from build123d import *

# Parameters (mm, degrees)
SKETCH_1_R      = 3
SKETCH_1_R_2    = 5
EXTRUDE_1_DEPTH = 5


# Read off the part's stored shape, not the designer's step: M5 螺纹孔1
with BuildPart() as part:
    # 草图1 → 凸台-拉伸1 (new, symmetric)
    with BuildSketch(Plane.XY):
        with BuildLine():
            Line((8.93988801, 1.038461538), (7.449906675, 13.865384615))
            ThreePointArc((7.449906675, 13.865384615), (0, 20.5), (-7.449906675, 13.865384615))
            Line((-7.449906675, 13.865384615), (-8.93988801, 1.038461538))
            ThreePointArc((-8.93988801, 1.038461538), (0, -9), (8.93988801, 1.038461538))
        make_face()
        with Locations((0, 13)):
            Circle(SKETCH_1_R, mode=Mode.SUBTRACT)
        Circle(SKETCH_1_R_2, mode=Mode.SUBTRACT)
    extrude(amount=EXTRUDE_1_DEPTH, both=True)

    # M5 螺纹孔1 outline → M5 螺纹孔1 (revolve, cut)
    with BuildSketch(Plane(origin=(0, 0, 0), x_dir=(0.707106781186549, 0.707106781186546, 0), z_dir=(0, 0, -1))):
        Polygon((2.1, -4.315295433), (2.1, -5.425), (2.525, -5), (2.525, -4.315295433), align=None)
        Polygon((2.1, -13.143744736), (2.1, -5.425), (2.1, -4.315295433), (0, -4.315295433), (0, -13.143744736), align=None)
    revolve(axis=Axis((0, 0, 0), (0.707106781186546, -0.707106781186549, 0)), mode=Mode.SUBTRACT)


solid = part.part
Build history of the part. All positions in model axes, mm. A direction names the side the tool comes from. Give positions to 0.01 mm unless a question says otherwise; leave off trailing zeros. Order: outer loops, then holes, each group sorted by start corner. A loop starts at its lowest first (then second) coordinate and runs counter-clockwise, first axis right, second up. Notation, with made-up numbers: M 37.25,27.25 L 88.25,27.25 A24 ccw 88.25,63.25 Z; hole C -29.5,5.5 d10. An arc over 180 degrees is marked long. Put each result on its own line as item: value.
Item 1: Probe line 1 (Y direction, x = -2.5, z = -1); line 2 (Y direction, x = 2.25, z = 1.75); line 3 (Z direction, x = -6.25, y = 6.5). List the from-to ranges inside material, lowest first. Write a range as [from, to].
From the geometry:
line 1: y = [-8.65, -4.33], [5.14, 11.34], [14.66, 20.07]
line 2: y = [-8.71, -4.47], [4.47, 11.02], [14.98, 20.15]
line 3: z = [-5, -2.09], [2.09, 5]
Item 2: Slice it at B-B, the plane y = 0. Write the cut outline in (x, z), plus the area to 3 significant figures.
From the geometry:
outline: M -9,-5 L -5,-5 L -5,5 L -9,5 Z; M 5,-5 L 9,-5 L 9,5 L 5,5 Z
area: 80.0 mm2
Item 3: Two-plate mould, pull along Y, no slides. Class faces 1 (the cylindrical face through (0.15, 20.5, 0.07)), 2 (the cylindrical face through (-5.13, 1.56, 0.06)), 3 (the flat face through (0, 6, 5)): +Y half, -Y half, draft (parallel to the pull), parting line (faces both ways), or undercut.
From the geometry:
face 1: +Y half
face 2: undercut
face 3: draft
Item 4: Slice it at D-D, the plane x = 7. Write the cut outline in (y, z), plus the area to 3 significant figures.
From the geometry:
outline: M -5.66,-5 L 15.69,-5 L 15.69,5 L -5.66,5 Z
area: 213 mm2
Item 5: Slice it at C-C, the plane y = 13. Write the cut outline in (x, z).
From the geometry:
outline: M -7.55,-5 L -3,-5 L -3,5 L -7.55,5 Z; M 3,-5 L 7.55,-5 L 7.55,5 L 3,5 Z
Item 6: 3-axis set-ups, long thin cutter, end or side, ignore diameter. For faces 4 (the flat face through (8.2, 7.4, 0.1)), 5 (the cylindrical face through (-1.56, 5.13, -0.06)): which of +Z, -Z, +X, -X, +Y, -Y reach the whole face in a straight line?
From the geometry:
face 4: +Z, -Z, +X, +Y
face 5: none
Item 7: Slice it at A-A, the plane x = 0. Write the cut outline in (y, z).
From the geometry:
outline: M -9,-5 L -5,-5 L -5,5 L -9,5 Z; M 5,-5 L 10,-5 L 10,5 L 5,5 Z; M 16,-5 L 20.5,-5 L 20.5,5 L 16,5 Z
Item 8: Flat gauge pins, fed straight in: pin 1 Ø8 at (x, y) = (0, 0) entering from -Z; pin 2 Ø3 at (x, z) = (-4, 0) entering from -Y; pin 3 Ø1 at (y, z) = (16.5, 0.5) entering from +X. Where does each tip first touch, or does it go through?
From the geometry:
pin 1: passes through
pin 2: stops at y = -8.65
pin 3: stops at x = 6.87
